Input: part model. Units: mm. Frame: model coordinates. A direction names the side the tool comes from. Round coordinates to 2 decimals unless told otherwise and drop trailing zeros. Order: outer loops, then holes, each group sorted by start corner. A loop starts at its lowest first (then second) coordinate and runs counter-clockwise, first axis right, second up. Notation, with made-up numbers: (48.25, 43) -> (84.25, 43) arc R12 ccw to (84.25, 52) -> close; hole circle Ø11 at (37.5, 76.5). An arc over 180 degrees is marked (long way). Use a Markdown table: item, result.
from build123d import *

# Parameters (mm, degrees)
SKETCH1_W           = 50
SKETCH1_H           = 50
BOSS_EXTRUDE1_DEPTH = 230
SKETCH2_W           = 30
SKETCH2_H           = 25
BOSS_EXTRUDE2_DEPTH = 10
SKETCH3_R           = 5
CUT_EXTRUDE1_DEPTH  = 100
SKETCH4_W           = 20
SKETCH4_H           = 20
CUT_EXTRUDE2_DEPTH  = 21
SKETCH5_R           = 1
CUT_EXTRUDE3_DEPTH  = 15


with BuildPart() as part:
    # Sketch1 → Boss-Extrude1 (new body)
    with BuildSketch(Plane(origin=(0, 0, 0), x_dir=(1, 0, 0), z_dir=(0, 1, 0))):
        Rectangle(SKETCH1_W, SKETCH1_H)
    extrude(amount=BOSS_EXTRUDE1_DEPTH)

    # Sketch2 → Boss-Extrude2 (add)
    with BuildSketch(Plane(origin=(0, 0, 0), x_dir=(-1, 0, 0), z_dir=(0, -1, 0))):
        Rectangle(SKETCH2_W, SKETCH2_H)
    extrude(amount=BOSS_EXTRUDE2_DEPTH)

    # Sketch3 → Cut-Extrude1 (cut)
    with BuildSketch(Plane(origin=(0, -10, 0), x_dir=(-1, 0, 0), z_dir=(0, -1, 0))):
        Circle(SKETCH3_R)
    extrude(amount=-CUT_EXTRUDE1_DEPTH, mode=Mode.SUBTRACT)

    # Sketch4 → Cut-Extrude2 (cut)
    with BuildSketch(Plane(origin=(0, 230, 0), x_dir=(1, 0, 0), z_dir=(0, 1, 0))):
        Rectangle(SKETCH4_W, SKETCH4_H)
    extrude(amount=-CUT_EXTRUDE2_DEPTH, mode=Mode.SUBTRACT)

    # Sketch5 → Cut-Extrude3 (cut)
    with BuildSketch(Plane.XY.offset(25)):
        with Locations((10, 200)):
            Circle(SKETCH5_R)
        with Locations((-10, 200)):
            Circle(SKETCH5_R)
    extrude(amount=-CUT_EXTRUDE3_DEPTH, mode=Mode.SUBTRACT)


solid = part.part
1) Draft query along X for faces 1 (the face through (0, -5, -12.5)), 2 (the face through (1.08, 39.3, 4.88)), 3 (the face through (15, -5, 0)). Return one class per face: released by +X, released by -X, zero draft, split by the parting line, or undercut.
Answer key:
| item | result |
|---|---|
| face 1 | zero draft |
| face 2 | undercut |
| face 3 | released by +X |
2) Cut plane C-C on z = 18. Return loops of the section in (x, y).
Answer key:
| item | result |
|---|---|
| outline | (-25, 0) -> (25, 0) -> (25, 230) -> (-25, 230) -> close; hole circle Ø2 at (-10, 200); hole circle Ø2 at (10, 200) |
3) Cut plane D-D on x = 0. Return loops of the section in (y, z), and give its area (3 significant figures).
Answer key:
| item | result |
|---|---|
| outline | (-10, -12.5) -> (0, -12.5) -> (0, -25) -> (230, -25) -> (230, -10) -> (209, -10) -> (209, 10) -> (230, 10) -> (230, 25) -> (0, 25) -> (0, 12.5) -> (-10, 12.5) -> (-10, 5) -> (90, 5) -> (90, -5) -> (-10, -5) -> close |
| area | 10,300 mm^2 |
4) Contact query for flat-ended pins moving along their axis: P1, Ø6, axis at x = 0, z = 0, coming from the -Y side; P2, Ø3, axis at y = -3, z = 6, coming from the -X side; P3, Ø3, axis at x = 10, y = 200, coming from the +Z side; P4, Ø5, axis at y = -6.5, z = -5.5, coming from the +X side. Output: stop coordinate, or through.
Answer key:
| item | result |
|---|---|
| P1 | stops at y = 90 |
| P2 | stops at x = -15 |
| P3 | stops at z = 25 |
| P4 | stops at x = 15 |
5) Set-up query: faces 4 (the face through (0, 220, 10)), 5 (the face through (0, 90, 0)), 6 (the face through (-15, -5, 0)). Return all of +Z, -Z, +X, -X, +Y, -Y with unobstructed straight access to the full face (end or side cutting, diameter ignored); none if empty.
Answer key:
| item | result |
|---|---|
| face 4 | +Y |
| face 5 | -Y |
| face 6 | +Z, -Z, -X, -Y |
6) Ray query, probe 1 along X at (y, z) = (200, 21); probe 2 along X at (y, z) = (44, 0); probe 3 along Y at (x, z) = (18.5, 21.5). Return the intervals inside material, ascending.
Answer key:
| item | result |
|---|---|
| probe 1 | x = -25 to -11, -9 to 9, 11 to 25 |
| probe 2 | x = -25 to -5, 5 to 25 |
| probe 3 | y = 0 to 230 |
7) Cut plane A-A on z = 0. Return loops of the section in (x, y), and give its area (3 significant figures).
Answer key:
| item | result |
|---|---|
| outline | (-25, 0) -> (-15, 0) -> (-15, -10) -> (-5, -10) -> (-5, 90) -> (5, 90) -> (5, -10) -> (15, -10) -> (15, 0) -> (25, 0) -> (25, 230) -> (10, 230) -> (10, 209) -> (-10, 209) -> (-10, 230) -> (-25, 230) -> close |
| area | 10,400 mm^2 |
8) Cut plane B-B on y = 38. Return loops of the section in (x, z), and give its area (3 significant figures).
Answer key:
| item | result |
|---|---|
| outline | (-25, -25) -> (25, -25) -> (25, 25) -> (-25, 25) -> close; hole circle Ø10 at (0, 0) |
| area | 2,420 mm^2 |
